Can you work these out from the model? Positions are in its coordinate system, mm. Face numbers are marked on the shaded views. A direction names the side the tool comes from. Give positions to 0.01 mm unless a question says otherwise; leave off trailing zeros. Loops run counter-clockwise (first coordinate to the right, second up) from the corner with the lowest first, then second, coordinate; pieces in that order, holes last. Notation, with made-up numbers: (75.5, 37.25) -> (101.5, 37.25) arc R19 cw to (101.5, 52.25) -> close; hole circle Ø11 at (2.5, -20.75). An arc over 180 degrees is marked (long way). Use CSV: the item, a comma, the result in double quotes.
Autodesk Inventor part; units mm, degrees
ref_plane "YZ Plane" through (0, 0, 0) normal (1, 0, 0) x (0, 1, 0)
ref_plane "XZ Plane" through (0, 0, 0) normal (0, 1, 0) x (-1, 0, 0)
ref_plane "XY Plane" through (0, 0, 0) normal (0, 0, 1) x (1, 0, 0)
sketch "Sketch1" plane through (0, 0, 0) normal (0, 0, 1) x (1, 0, 0)
  circle A0 centre (0, 0) radius 26.054
  circle A1 centre (0, 0) radius 69.55
  circle A2 centre (0, 53.975) radius 3.3734
  circle A3 centre (-46.7437, 26.9875) radius 3.3734
  circle A4 centre (-46.7437, -26.9875) radius 3.3734
  circle A5 centre (0, -53.975) radius 3.3734
  circle A6 centre (46.7437, -26.9875) radius 3.3734
  circle A7 centre (46.7437, 26.9875) radius 3.3734
  dimension "d0" = 52.108
  dimension "d1" = 139.1
  dimension "d2" = 6.7469
  dimension "d3" = 53.975
  dimension "d6" = 360
extrude "Extrusion1" add sketch "Sketch1" along normal blind 12.7
sketch "Sketch2" plane through (0, 0, 12.7) normal (0, 0, 1) x (1, 0, 0)
  circle A0 centre (0, 0) radius 38.1
  circle A1 centre (0, 0) radius 26.054
  dimension "d10" = 76.2
extrude "Extrusion2" add sketch "Sketch2" along normal blind 50.8
chamfer "Chamfer1" distance 6.35 distance2 41.275 1 edges at (-38.1, 0, 63.5) measured on face at (33.7663, -2.826, 63.5)
chamfer "Chamfer2" distance 0.508 angle 45 4 edges at (-69.55, 0, 12.7) (-69.55, 0, 0) (-26.054, 0, 0) (-26.054, 0, 63.5)
properties part number "ExtendedIndexerPivot"
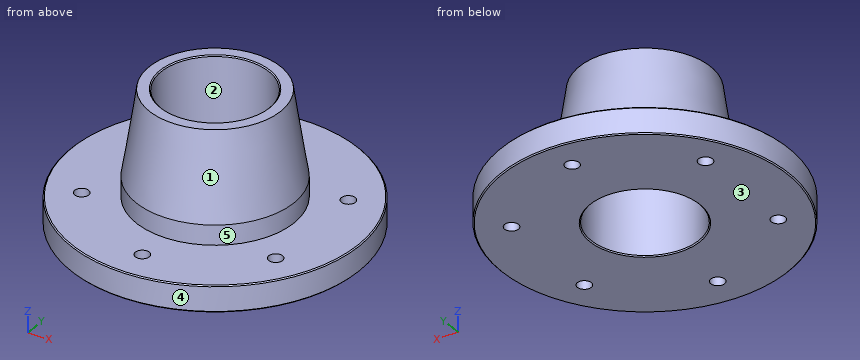
(1) If we section it at C-C, the plane z = 20: Write out the boundary of the cut face in (x, y).
Answer sheet:
outline,"circle Ø76.2 at (0, 0); hole circle Ø52.11 at (0, 0)"
(2) We'd pull the mould along X, two halves only. Please class the marked faces 1, 2 and 3: released by +X, released by -X, zero draft, split by the parting line, or undercut.
Answer sheet:
face 1,"split by the parting line"
face 2,"undercut"
face 3,"zero draft"
(3) If we section it at B-B, the plane x = 0: Give the number of separate pieces and of enclosed holes in the cut face, then the cut area to 3 significant figures.
Answer sheet:
separate pieces,"4"
enclosed holes,"0"
area,"1,890 mm2"
(4) Will these pins go through, and if not, where does the flat tip stop? pin 1 Ø5.5 at (x, y) = (46.74, -26.99) entering from +Z; pin 2 Ø3 at (x, y) = (-10, -54) entering from +Z; pin 3 Ø10 at (x, z) = (27.5, 50.5) entering from +Y; pin 4 Ø9 at (x, y) = (-46.74, -26.99) entering from -Z.
Answer sheet:
pin 1,"passes through"
pin 2,"stops at z = 12.7"
pin 3,"stops at y = 25.27"
pin 4,"stops at z = 0"
(5) If we section it at A-A, the plane y = 0: Write out the boundary of the cut face in (x, z) (3 decimals).
Answer sheet:
outline,"(-69.55, 0.508) -> (-69.042, 0) -> (-26.562, 0) -> (-26.054, 0.508) -> (-26.054, 62.992) -> (-26.562, 63.5) -> (-31.75, 63.5) -> (-38.1, 22.225) -> (-38.1, 12.7) -> (-69.042, 12.7) -> (-69.55, 12.192) -> close; (26.054, 0.508) -> (26.562, 0) -> (69.042, 0) -> (69.55, 0.508) -> (69.55, 12.192) -> (69.042, 12.7) -> (38.1, 12.7) -> (38.1, 22.225) -> (31.75, 63.5) -> (26.562, 63.5) -> (26.054, 62.992) -> close"
(6) Which directions (+Z, -Z, +X, -X, +Y, -Y) give clear straight access to the entire face, cutting with the end or side of a thin tool? Please do the marked faces 4 and 5.
Answer sheet:
face 4,"+Z, -Z"
face 5,"+Z"
(7) If I drill on L1, parallel to Y at x = 0, z = 8; L2, parallel to Z at x = 40.5, y = -0.5; L3, parallel to X at y = -9, z = 55.5, over which ranges is the centre line in solid material (lowest first)? Write a range as from..to.
Answer sheet:
L1,"y = -69.55..-57.35, -50.6..-26.05, 26.05..50.6, 57.35..69.55"
L2,"z = 0..12.7"
L3,"x = -31.73..-24.45, 24.45..31.73"
(8) If we section it at D-D, the plane z = 39.5: Write out the boundary of the cut face in (x, y).
Answer sheet:
outline,"circle Ø70.88 at (0, 0); hole circle Ø52.11 at (0, 0)"
